Here's how the part is built. I have some questions about the finished solid (model axes, mm). Face numbers are marked on the shaded views. Round coordinates to 2 decimals unless told otherwise and drop trailing zeros. Write each loop counter-clockwise with the first axis right and the second up, starting at its lowest first coordinate (ties: lowest second). Pieces come first, ordered by that corner, then holes. Notation, with made-up numbers: (68.25, -2) -> (78.25, -2) arc R23 ccw to (78.25, 28) -> close; hole circle Ø11 at (10.25, 3.5). An arc over 180 degrees is marked (long way). Answer in a Markdown table with one row per item.
from build123d import *

# Parameters (mm, degrees)
SKETCH1_R             = 35
BOSS_EXTRUDE1_DEPTH   = 15
CUT_EXTRUDE1_REACH    = 53.72
SKETCH2_R             = 5
SKETCH3_R             = 6.5
CUT_EXTRUDE2_DEPTH    = 5
CUT_EXTRUDE3_REACH    = 53.72
SKETCH4_R             = 2.05
M6_CLEARANCE_HOLE1_D  = 6.4
F_8_0MM_DOWEL_HOLE1_D = 8
CHAMFER1_SIZE         = 0.5


with BuildPart() as part:
    # Sketch1 → Boss-Extrude1 (new body)
    with BuildSketch(Plane(origin=(0, 0, 0), x_dir=(1, 0, 0), z_dir=(0, 1, 0))):
        with Locations(Location((0, 0, 0), (0, 0, 270))):
            Circle(SKETCH1_R)
    extrude(amount=BOSS_EXTRUDE1_DEPTH)

    # Sketch2 → Cut-Extrude1 (cut, up to next)
    with BuildSketch(Plane(origin=(0, 15, 0), x_dir=(1, 0, 0), z_dir=(0, 1, 0)), mode=Mode.PRIVATE) as cut_extrude1_sk1:
        with Locations(Location((0, 0, 0), (0, 0, 270))):
            Circle(SKETCH2_R)
    cut_extrude1_tool1 = extrude(cut_extrude1_sk1.sketch, amount=-CUT_EXTRUDE1_REACH, mode=Mode.PRIVATE) & part.part
    add(cut_extrude1_tool1.solids().sort_by_distance((0, 15, 0))[0], mode=Mode.SUBTRACT)

    # Sketch3 → Cut-Extrude2 (cut)
    with BuildSketch(Plane(origin=(0, 15, 0), x_dir=(1, 0, 0), z_dir=(0, 1, 0))):
        with Locations(Location((0, 0, 0), (0, 0, 270))):
            Circle(SKETCH3_R)
    extrude(amount=-CUT_EXTRUDE2_DEPTH, mode=Mode.SUBTRACT)

    # Sketch4 → Cut-Extrude3 (cut, up to next)
    with BuildSketch(Plane(origin=(0, 15, 0), x_dir=(1, 0, 0), z_dir=(0, 1, 0)), mode=Mode.PRIVATE) as cut_extrude3_sk1:
        with Locations(Location((0, 10, 0), (0, 0, 270))):
            Circle(SKETCH4_R)
    cut_extrude3_tool1 = extrude(cut_extrude3_sk1.sketch, amount=-CUT_EXTRUDE3_REACH, mode=Mode.PRIVATE) & part.part
    # Sketch4 → Cut-Extrude3 (cut, up to next)
    with BuildSketch(Plane(origin=(0, 15, 0), x_dir=(1, 0, 0), z_dir=(0, 1, 0)), mode=Mode.PRIVATE) as cut_extrude3_sk2:
        with Locations(Location((8.660254038, -5, 0), (0, 0, 270))):
            Circle(SKETCH4_R)
    cut_extrude3_tool2 = extrude(cut_extrude3_sk2.sketch, amount=-CUT_EXTRUDE3_REACH, mode=Mode.PRIVATE) & part.part
    # Sketch4 → Cut-Extrude3 (cut, up to next)
    with BuildSketch(Plane(origin=(0, 15, 0), x_dir=(1, 0, 0), z_dir=(0, 1, 0)), mode=Mode.PRIVATE) as cut_extrude3_sk3:
        with Locations(Location((-8.660254038, -5, 0), (0, 0, 270))):
            Circle(SKETCH4_R)
    cut_extrude3_tool3 = extrude(cut_extrude3_sk3.sketch, amount=-CUT_EXTRUDE3_REACH, mode=Mode.PRIVATE) & part.part
    add(cut_extrude3_tool1.solids().sort_by_distance((0, 15, -10))[0], mode=Mode.SUBTRACT)
    add(cut_extrude3_tool2.solids().sort_by_distance((8.660254, 15, 5))[0], mode=Mode.SUBTRACT)
    add(cut_extrude3_tool3.solids().sort_by_distance((-8.660254, 15, 5))[0], mode=Mode.SUBTRACT)

    # M6 Clearance Hole1 (through all)
    with Locations(Plane(origin=(0, 0, 0), x_dir=(-1, 0, 0), z_dir=(0, -1, 0))):
        with Locations((0, 25), (21.650635095, -12.5), (-21.650635095, -12.5)):
            Hole(M6_CLEARANCE_HOLE1_D / 2)

    # Ø8.0mm Dowel Hole1 (through all)
    with Locations(Plane(origin=(0, 0, 0), x_dir=(-1, 0, 0), z_dir=(0, -1, 0))):
        with Locations((-13.75, 23.815698604), (13.75, -23.815698604)):
            Hole(F_8_0MM_DOWEL_HOLE1_D / 2)

    # Chamfer1
    chamfer1_edges = [part.edges().sort_by_distance(p)[0] for p in [
        (0, 0, -35),
        (0, 15, -35),
    ]]
    chamfer(chamfer1_edges, length=CHAMFER1_SIZE)


solid = part.part
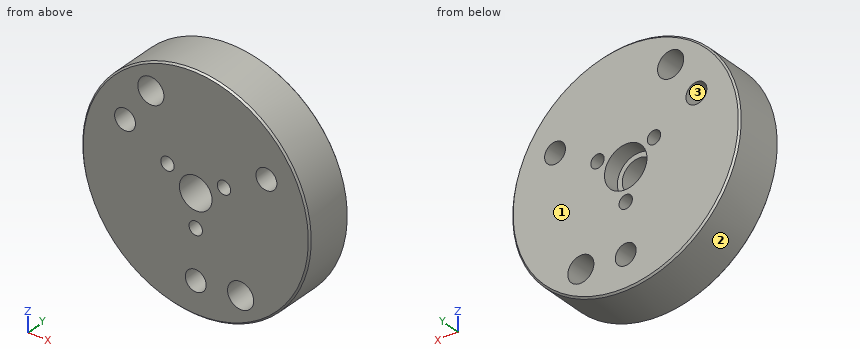
1) For pin 1 (3 mm diameter, centred on x = -10, y = 10, fed in from -Z); pin 2 (8 mm diameter, centred on y = 2.5, z = 3.5, fed in from +X); pin 3 (5 mm diameter, centred on y = 13.5, z = -9, fed in from -X), each with a flat end and sliding along its axis, tell me the tip position at first contact or that it passes through.
Response:
| item | result |
|---|---|
| pin 1 | stops at z = -33.95 |
| pin 2 | stops at x = 35 |
| pin 3 | stops at x = -34.39 |
2) We'd pull the mould along Z, two halves only. Please class the marked faces 1, 2 and 3: +Z half, -Z half, draft (parallel to the pull), parting line (faces both ways), or undercut.
Response:
| item | result |
|---|---|
| face 1 | draft |
| face 2 | parting line |
| face 3 | undercut |
3) I want a section at C-C, the plane y = 7.75. Count the separate pieces of the cut face and the enclosed holes in it, and give its area (3 significant figures).
Response:
| item | result |
|---|---|
| separate pieces | 1 |
| enclosed holes | 9 |
| area | 3,530 mm^2 |
4) I need wall thicknesses on line 1 (X direction, y = 3, z = 0); line 2 (X direction, y = 12.4, z = 0); line 3 (Z direction, x = 13.75, y = 9.75). Which ranges of each line are inside material? Lowest first, please. Write a range as [from, to].
Response:
| item | result |
|---|---|
| line 1 | x = [-35, -5], [5, 35] |
| line 2 | x = [-35, -6.5], [6.5, 35] |
| line 3 | z = [-32.19, -27.82], [-19.82, 32.19] |
5) I want a section at B-B, the plane x = 0. List the corners of the cut face in (y, z) for me, and give its area (3 significant figures).
Response:
| item | result |
|---|---|
| outline | (0, -34.5) -> (0.5, -35) -> (14.5, -35) -> (15, -34.5) -> (15, -28.2) -> (0, -28.2) -> close; (0, -21.8) -> (15, -21.8) -> (15, -12.05) -> (0, -12.05) -> close; (0, -7.95) -> (15, -7.95) -> (15, -6.5) -> (10, -6.5) -> (10, -5) -> (0, -5) -> close; (0, 5) -> (10, 5) -> (10, 6.5) -> (15, 6.5) -> (15, 34.5) -> (14.5, 35) -> (0.5, 35) -> (0, 34.5) -> close |
| area | 727 mm^2 |
6) I want a section at A-A, the plane z = 0. List the corners of the cut face in (x, y) for me.
Response:
| item | result |
|---|---|
| outline | (-35, 0.5) -> (-34.5, 0) -> (-5, 0) -> (-5, 10) -> (-6.5, 10) -> (-6.5, 15) -> (-34.5, 15) -> (-35, 14.5) -> close; (5, 0) -> (34.5, 0) -> (35, 0.5) -> (35, 14.5) -> (34.5, 15) -> (6.5, 15) -> (6.5, 10) -> (5, 10) -> close |
